Work out the finished part from the listing and answer in its coordinate system (mm). A direction names the side the tool comes from. Coordinates: 2 decimals unless noted, no trailing zeros. Write each loop counter-clockwise with the first axis right and the second up, starting at its lowest first coordinate (ties: lowest second). Pieces come first, ordered by that corner, then holes. Notation, with made-up numbers: (30, 14.5) - (89, 14.5) arc R20 ccw to (89, 31.5) - close; hole circle Ø7 at (53.25, 67.25). An arc over 180 degrees is marked (long way). One line per item, written item: value.
```python
from build123d import *

# Parameters (mm, degrees)
EXTRUDE_1_DEPTH             = 10
FILLET_1_R                  = 0.3
FILLET_2_R                  = 2
HOLE_WIZARD_M81_D           = 6.8
HOLE_WIZARD_M81_CSINK_D     = 8.05
HOLE_WIZARD_M81_CSINK_ANGLE = 90


with BuildPart() as part:
    # Эскиз1 → Бобышка-Вытянуть1 (new body, symmetric)
    with BuildSketch(Plane.XY):
        with BuildLine():
            Line((-4, 0), (4, 0))
            Line((4, 0), (4, -0.8))
            Line((4, -0.8), (6, -0.8))
            Line((6, -0.8), (6, -1.6))
            ThreePointArc((6, -1.6), (4.120585945, -4.832650297), (1.5, -7.5))
            Line((1.5, -7.5), (-1.5, -7.5))
            ThreePointArc((-1.5, -7.5), (-4.120585945, -4.832650297), (-6, -1.6))
            Line((-6, -1.6), (-6, -0.8))
            Line((-6, -0.8), (-4, -0.8))
            Line((-4, -0.8), (-4, 0))
        make_face()
    extrude(amount=EXTRUDE_1_DEPTH, both=True)

    # Скругление1
    fillet_1_edges = [part.edges().sort_by_distance(p)[0] for p in [
        (6, -0.8, 0),
        (6, -1.6, 0),
        (-6, -1.6, 0),
        (-6, -0.8, 0),
        (-4, 0, 0),
        (4, 0, 0),
    ]]
    fillet(fillet_1_edges, radius=FILLET_1_R)

    # Скругление2
    fillet_2_edges = [part.edges().sort_by_distance(p)[0] for p in [
        (1.5, -7.5, 0),
        (-1.5, -7.5, 0),
    ]]
    fillet(fillet_2_edges, radius=FILLET_2_R)

    # Отверстие обработанное метчиком M81 (through all)
    with Locations(Plane(origin=(0, 0, 0), x_dir=(1, 0, 0), z_dir=(0, 1, 0))):
        with Locations((0, -4)):
            CounterSinkHole(HOLE_WIZARD_M81_D / 2, HOLE_WIZARD_M81_CSINK_D / 2, counter_sink_angle=HOLE_WIZARD_M81_CSINK_ANGLE)

    # Эскиз5 → Повернуть1 (revolve)
    with BuildSketch(Plane(origin=(0, 0, 0), x_dir=(0, 0, -1), z_dir=(1, 0, 0))):
        with BuildLine():
            Line((6, -4.3), (6, -8.3))
            ThreePointArc((6, -8.3), (4, -6.3), (6, -4.3))
        make_face()
    revolve(axis=Axis((0, -4.3, -6), (0, -1, 0)))


solid = part.part
```
Item 1: Section B-B, the plane z = 4 is taken. Determine the outline of the cut face in (x, y) (3 decimals), then the cut area to 3 significant figures.
Evaluation:
outline: (-6, -1.539) arc R0.3 ccw to (-5.976, -1.657) arc R15 ccw to (-3.4, -5.707) - (-3.4, -0.625) - (-3.924, -0.101) arc R0.3 ccw to (-4, -0.3) - (-4, -0.8) - (-5.7, -0.8) arc R0.3 ccw to (-6, -1.1) - close; (3.4, -5.707) arc R15 ccw to (5.976, -1.657) arc R0.3 ccw to (6, -1.539) - (6, -1.1) arc R0.3 ccw to (5.7, -0.8) - (4, -0.8) - (4, -0.3) arc R0.3 ccw to (3.924, -0.101) - (3.4, -0.625) - close
area: 16.6 mm2
Item 2: Which of the six approach directions +Z, -Z, +X, -X, +Y, -Y give full straight-line access (tool end or side, diameter ignored) to faces 5 (the face through (-1.49, -7.37, -4.42)), 6 (the face through (0, -7.5, 9)), 7 (the face through (-5, -0.8, 0)), 8 (the face through (1.49, -7.37, 8.31))?
Evaluation:
face 5: -X, -Y
face 6: +Z, +X, -X, -Y
face 7: +Z, -Z, -X, +Y
face 8: +Z, +X, -Y
Item 3: Consider probe 1 along Z at (x, y) = (0, -2.75); probe 2 along Z at (x, y) = (2.25, -5.5); probe 3 along X at (y, z) = (-4.75, 4.25). Determine where each line is inside the solid, lowest interval first.
Evaluation:
probe 1: z = -10 to 0.6, 7.4 to 10
probe 2: z = -10 to 1.45, 6.55 to 10
probe 3: x = -4.18 to -3.39, 3.39 to 4.18
Item 4: Section D-D, the plane x = 5 is taken. Determine the outline of the cut face in (y, z).
Evaluation:
outline: (-3.55, -10) - (-0.8, -10) - (-0.8, 10) - (-3.55, 10) - close
Item 5: Determine the mould class of faces 1 (the face through (0, -7.5, -2)), 2 (the face through (-1.49, -7.37, 8.31)), 3 (the face through (1.49, -7.37, -4.42)), 4 (the face through (3.4, -4.1, 3.9)) for opening direction X: +X half, -X half, draft (parallel to the pull), parting line (faces both ways), or undercut.
Evaluation:
face 1: draft
face 2: -X half
face 3: +X half
face 4: undercut
Item 6: Section C-C, the plane y = -3.25 is taken. Determine the outline of the cut face in (x, z), then the cut area to 3 significant figures.
Evaluation:
outline: (-5.18, -10) - (5.18, -10) - (5.18, 10) - (-5.18, 10) - close; hole circle Ø6.8 at (0, 4)
area: 171 mm2
Item 7: Given pin 1 (1.7 mm diameter, centred on x = -0.5, z = 8, fed in from -Y); pin 2 (1.9 mm diameter, centred on x = 5, z = -2.5, fed in from +Y); pin 3 (6 mm diameter, centred on x = 0, z = 5, fed in from +Y) (3 decimals); pin 4 (1 mm diameter, centred on y = -6.5, z = 4.5, fed in from -X), each flat-ended and moving along its own axis, determine where each tip first touches the part or whether it passes through.
Evaluation:
pin 1: stops at y = -7.5
pin 2: stops at y = -0.8
pin 3: stops at y = -0.025
pin 4: passes through
Item 8: Section A-A, the plane x = 0 is taken. Determine the outline of the cut face in (y, z) (3 decimals).
Evaluation:
outline: (-7.5, -10) - (0, -10) - (0, -0.025) - (-0.625, 0.6) - (-7.5, 0.6) - (-7.5, -4.4) arc R2 ccw to (-7.5, -7.6) - close; (-7.5, 7.4) - (-0.625, 7.4) - (0, 8.025) - (0, 10) - (-7.5, 10) - close
